```python
from build123d import *

# Parameters (mm, degrees)
BOSS_EXTRUDE1_DEPTH            = 1.6
F_2_2_2_2_DIAMETER_HOLE1_D     = 2.2
F_2_2_2_2_DIAMETER_HOLE1_DEPTH = 5
SKETCH8_W                      = 82.4
SKETCH8_H                      = 0.2
SKETCH8_W_2                    = 0.2
SKETCH8_H_2                    = 82.4
EXTRUDE1_DEPTH                 = 2.6


with BuildPart() as part:
    # Sketch1 → Boss-Extrude1 (new body)
    with BuildSketch(Plane(origin=(0, 0, 0), x_dir=(1, 0, 0), z_dir=(0, 1, 0))):
        Polygon((-34.144384454, 27.628503563), (-27.144384454, 27.628503563), (-27.144384454, 34.628503563), (55.255615546, 34.628503563), (55.255615546, 27.628503563), (62.255615546, 27.628503563), (62.255615546, -54.771496437), (55.255615546, -54.771496437), (55.255615546, -61.771496437), (-27.144384454, -61.771496437), (-27.144384454, -54.771496437), (-34.144384454, -54.771496437), align=None)
    extrude(amount=BOSS_EXTRUDE1_DEPTH)

    # Ø2.2 (2.2) Diameter Hole1
    with Locations(Plane(origin=(0, 1.6, 0), x_dir=(1, 0, 0), z_dir=(0, 1, 0))):
        with Locations((14.055615546, 32.628503563), (14.055615546, -59.771496437), (-32.144384454, -51.071496437), (60.255615546, 23.928503563), (-32.144384454, 23.928503563), (60.255615546, -51.071496437)):
            Hole(F_2_2_2_2_DIAMETER_HOLE1_D / 2, depth=F_2_2_2_2_DIAMETER_HOLE1_DEPTH)

    # Sketch8 → Extrude1 (cut, through all)
    with BuildSketch(Plane(origin=(0, 1.6, 0), x_dir=(1, 0, 0), z_dir=(0, 1, 0))):
        with Locations((14.055615546, 34.528503563)):
            Rectangle(SKETCH8_W, SKETCH8_H)
        with Locations((62.155615546, -13.571496437)):
            Rectangle(SKETCH8_W_2, SKETCH8_H_2)
        with Locations((14.055615546, -61.671496437)):
            Rectangle(SKETCH8_W, SKETCH8_H)
        with Locations((-34.044384454, -13.571496437)):
            Rectangle(SKETCH8_W_2, SKETCH8_H_2)
    extrude(amount=-EXTRUDE1_DEPTH, mode=Mode.SUBTRACT)


solid = part.part
```
Design review of the part built by this model. Coordinates are the model's own, in mm. Coordinates: 2 decimals unless noted, no trailing zeros. Loops run counter-clockwise (first coordinate to the right, second up) from the corner with the lowest first, then second, coordinate; pieces in that order, holes last. Notation, with made-up numbers: (43, 40) -> (82, 40) arc R26 ccw to (82, 63) -> close; hole circle Ø2 at (49, 35). An arc over 180 degrees is marked (long way). Answer as a JSON object with one key per item and string values.
Q1. Clearance check with flat-ended pins moving along their axes: pin 1 Ø0.8 at (x, y) = (-30.5, 1) entering from +Z; pin 2 Ø0.5 at (y, z) = (0.5, 58) entering from +X; pin 3 Ø0.5 at (y, z) = (1, 59.5) entering from -X. State where each tip first meets the part, or that it passes through.
Answer block:
{"pin 1": "stops at z = 54.77", "pin 2": "stops at x = 55.26", "pin 3": "stops at x = -27.14"}
Q2. Take a section at A-A on y = 0.6. Give the boundary of the cut face in (x, z).
Answer block:
{"outline": "(-33.94, -27.63) -> (-27.14, -27.63) -> (-27.14, -34.43) -> (55.26, -34.43) -> (55.26, -27.63) -> (62.06, -27.63) -> (62.06, 54.77) -> (55.26, 54.77) -> (55.26, 61.57) -> (-27.14, 61.57) -> (-27.14, 54.77) -> (-33.94, 54.77) -> close; hole circle Ø2.2 at (-32.14, -23.93); hole circle Ø2.2 at (-32.14, 51.07); hole circle Ø2.2 at (14.06, -32.63); hole circle Ø2.2 at (14.06, 59.77); hole circle Ø2.2 at (60.26, -23.93); hole circle Ø2.2 at (60.26, 51.07)"}
Q3. To check wall thickness, follow L1, parallel to Z at x = 14, y = 0.95; L2, parallel to Z at x = 14.5, y = 0.2. State the ranges of each line that lie inside material, in increasing order.
Answer block:
{"L1": "z = -34.43 to -33.73, -31.53 to 58.67, 60.87 to 61.57", "L2": "z = -34.43 to -33.63, -31.62 to 58.77, 60.78 to 61.57"}
Q4. The part is to be moulded in two halves that separate along X. For faces 1 (the cylindrical face through (59.24, 0.79, -23.51)), 2 (the flat face through (15, 1.6, 13)), say which applies: +X half, -X half, draft (parallel to the pull), parting line (faces both ways), or undercut.
Answer block:
{"face 1": "undercut", "face 2": "draft"}
